Read the model definition and answer for the solid it produces. Units are mm, in the model's axes. A direction names the side the tool comes from. Round coordinates to 2 decimals unless told otherwise and drop trailing zeros. Use one line per item in the form item = value. Start each with the question number.
```python
from build123d import *

# Parameters (mm, degrees)
F0_W     = 30
F0_H     = 30
F1_DEPTH = 5
F2_W     = 5
F2_H     = 35
F3_DEPTH = 30
F4_R     = 1.625
F5_DEPTH = 25
F6_R     = 4.99999
F7_R     = 3
F8_DEPTH = 25
F9_R     = 4.99999


# Not quite as in the source:
# - a fillet or chamfer is up to 0.001 mm smaller than in the source, because OpenCascade refuses the exact size


with BuildPart() as f1:
    # F0 (on Top) → F1 (new body)
    with BuildSketch(Plane.XY):
        with Locations((0, 15)):
            Rectangle(F0_W, F0_H)
    extrude(amount=F1_DEPTH)

    # F2 (on face) → F3 (join)
    with BuildSketch(Plane.YZ.offset(15)):
        with Locations((2.5, 22.5)):
            Rectangle(F2_W, F2_H)
    extrude(amount=-F3_DEPTH)

    # F4 (on face) → F5 (cut)
    with BuildSketch(Plane.XY.offset(5)):
        with Locations((0, 17.5)):
            Circle(F4_R)
    extrude(amount=-F5_DEPTH, mode=Mode.SUBTRACT)

    # F6 (radius 5 in the source; OpenCascade refuses exactly that, so slightly less here)
    f6_edges = [f1.edges().sort_by_distance(p)[0] for p in [
        (0, 30, 5),
        (15, 17.5, 5),
        (-15, 17.5, 5),
        (15, 30, 2.5),
        (-15, 30, 2.5),
    ]]
    fillet(f6_edges, radius=F6_R)

    # F7 (on face) → F8 (cut)
    with BuildSketch(Plane.XZ):
        with Locations((0, 30)):
            Circle(F7_R)
        with Locations((0, 20.5)):
            Circle(F7_R)
    extrude(amount=-F8_DEPTH, mode=Mode.SUBTRACT)

    # F9 (radius 5 in the source; OpenCascade refuses exactly that, so slightly less here)
    f9_edges = [f1.edges().sort_by_distance(p)[0] for p in [
        (15, 5, 20.000005),
        (-15, 5, 20.000005),
        (0, 5, 40),
        (15, 2.5, 40),
        (-15, 2.5, 40),
    ]]
    fillet(f9_edges, radius=F9_R)


solid = f1.part
```
Q1. For a pull along X with two mould halves and no side action, classify faces 6 (the face through (-2.21, 2.46, 32.03)), 7 (the face through (0, 4, 38)), 8 (the face through (-0.352, 15.914, 2.535)), 9 (the face through (14, 3, 18)) as +X half, -X half, draft (parallel to the pull), parting line (faces both ways), or undercut.
Q2. Each of these flat-tipped pins is pushed along its axis until it touches: pin 1 Ø5 at (x, y) = (0, 17.5) entering from +Z; pin 2 Ø6 at (y, z) = (5.5, 32) entering from +X; pin 3 Ø1.5 at (x, y) = (-4, 26.5) entering from -Z; pin 4 Ø7 at (x, z) = (0, 20.5) entering from +Y. Where does it stop, or does it pass through?
Q3. Find section A-A on x = 0. Count the separate pieces of the cut face and the enclosed holes in it, and give its area (3 significant figures).
Q4. Straight lines are drawn through the part: line 1 (Z direction, x = 0, y = 1.15); line 2 (Y direction, x = -10, z = 15). For each, find the intervals that lie inside material, in ascending order. Write a range as [from, to].
Q5. A tool of negligible diameter and unlimited length cuts with its end or side. For faces 1 (the face through (-14, 15, 3)), 2 (the face through (14, 15, 3)), 3 (the face through (0, 15, 0)), 4 (the face through (0, 15, 5)), 5 (the face through (-0.65, 2.46, 17.57)), from which of +Z, -Z, +X, -X, +Y, -Y can it reach the whole face along a straight path? Write none if from no direction.
Response:
q1.face_6 = undercut
q1.face_7 = draft
q1.face_8 = undercut
q1.face_9 = +X half
q2.pin_1 = 5
q2.pin_2 = 14.33
q2.pin_3 = 0
q2.pin_4 = 5
q3.separate_pieces = 4
q3.enclosed_holes = 0
q3.area = 238 mm²
q4.line_1 = [0, 17.5], [23.5, 27], [33, 39.87]
q4.line_2 = [0, 5]
q5.face_1 = +Z, -X, +Y
q5.face_2 = +Z, +X, +Y
q5.face_3 = -Z, +X, -X, +Y, -Y
q5.face_4 = +Z, +X, -X, +Y
q5.face_5 = +Y, -Y
